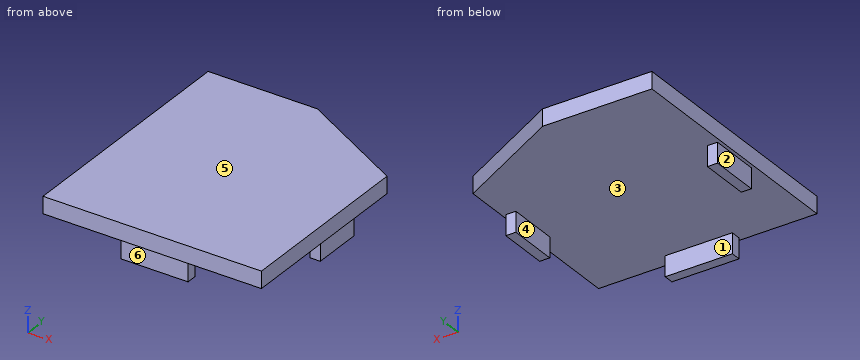
Autodesk Inventor part; units mm, degrees
ref_plane "YZ Plane" through (0, 0, 0) normal (1, 0, 0) x (0, 1, 0)
ref_plane "XZ Plane" through (0, 0, 0) normal (0, 1, 0) x (-1, 0, 0)
ref_plane "XY Plane" through (0, 0, 0) normal (0, 0, 1) x (1, 0, 0)
sketch "Sketch1" plane through (0, 0, 0) normal (0, 0, 1) x (1, 0, 0)
  line L0 (0, 175.2) -> (0, -29.2)
  line L1 (-91, 0) -> (91, 0)
  line L2 (0, 0) -> (-65, 0)
  line L3 (-65, 0) -> (-65, 146)
  line L4 (0, 0) -> (65, 0)
  line L5 (65, 0) -> (65, 111)
  line L6 (-65, 146) -> (0, 146)
  line L7 (0, 146) -> (65, 111)
  dimension "d0" = 65
  dimension "d1" = 146
  dimension "d2" = 65
  dimension "d3" = 111
  dimension "d4" = 65
extrude "Extrusion1" add sketch "Sketch1" along normal blind 10
sketch "Sketch2" plane through (0, 0, 0) normal (0, 0, -1) x (-1, 0, 0)
  line L0 (0, -29.2) -> (0, 175.2)
  line L1 (-91, 0) -> (91, 0)
  line L2 (65, 146) -> (65, 0)
  line L3 (0, 146) -> (65, 146)
  line L4 (-65, 111) -> (0, 146)
  line L5 (-65, 0) -> (-65, 111)
  line L6 (65, 0) -> (-65, 0)
  line L7 (-65, 0) -> (-55, 0)
  line L8 (-55, 0) -> (-55, 116.3846)
  line L9 (65, 0) -> (65, 10)
  line L10 (65, 10) -> (-65, 10)
  line L11 (65, 0) -> (55, 0)
  line L12 (55, 0) -> (55, 146)
  line L13 (-65, 0) -> (-65, 70)
  line L14 (-65, 70) -> (-63, 70)
  line L15 (-63, 70) -> (-63, 85)
  line L16 (-63, 85) -> (-57, 85)
  line L17 (-57, 85) -> (-57, 55)
  line L18 (-57, 55) -> (-63, 55)
  line L19 (-63, 55) -> (-63, 70)
  line L20 (65, 0) -> (65, 70)
  line L21 (65, 70) -> (63, 70)
  line L22 (63, 70) -> (63, 85)
  line L23 (63, 85) -> (57, 85)
  line L24 (57, 85) -> (57, 55)
  line L25 (57, 55) -> (63, 55)
  line L26 (63, 70) -> (63, 55)
  line L27 (0, 0) -> (0, 2)
  line L28 (0, 2) -> (-20, 2)
  line L29 (-20, 2) -> (-20, 8)
  line L30 (-20, 8) -> (20, 8)
  line L31 (20, 8) -> (20, 2)
  line L32 (20, 2) -> (0, 2)
  dimension "d7" = 10
  dimension "d8" = 10
  dimension "d9" = 10
  dimension "d10" = 70
  dimension "d11" = 2
  dimension "d12" = 15
  dimension "d13" = 6
  dimension "d14" = 30
  dimension "d15" = 70
  dimension "d16" = 2
  dimension "d17" = 15
  dimension "d18" = 6
  dimension "d19" = 30
  dimension "d20" = 2
  dimension "d21" = 20
  dimension "d22" = 6
  dimension "d23" = 40
extrude "Extrusion2" add sketch "Sketch2" along normal blind 12 contours L28 L29 L30 L0 | L0 L30 L31 L32 | L15 L16 L17 L18 L19 | L26 L25 L24 L23 L22
properties part number "Afsluitklep"
Could you check a few things on this model? Use its own coordinates, in mm. Face numbers are marked on the shaded views. A direction names the side the tool comes from. Give positions to 0.01 mm unless a question says otherwise; leave off trailing zeros. Loops run counter-clockwise (first coordinate to the right, second up) from the corner with the lowest first, then second, coordinate; pieces in that order, holes last. Notation, with made-up numbers: (47, 27.5) - (98, 27.5) arc R11 ccw to (98, 39.5) - close; hole circle Ø3 at (6.25, -23). An arc over 180 degrees is marked (long way). Answer in a Markdown table with one row per item. Add a question column.
Q1. If we section it at C-C (y = 73.5): List the corners of the cut face in (x, z) for me.
Q2. For pin 1 (1.5 mm diameter, centred on x = 29, y = 68.5, fed in from -Z); pin 2 (6 mm diameter, centred on y = 63.5, z = -6, fed in from -X); pin 3 (6 mm diameter, centred on y = 72.5, z = -5.5, fed in from +X); pin 4 (2 mm diameter, centred on x = -24, z = 3, fed in from -Y), each with a flat end and sliding along its axis, tell me the tip position at first contact or that it passes through.
Q3. We'd pull the mould along X, two halves only. Please class the marked faces 1, 2 and 3: +X half, -X half, draft (parallel to the pull), parting line (faces both ways), or undercut.
Q4. Please list where these lines run through material, in increasing order: L1, parallel to Z at x = 1, y = 62.5; L2, parallel to X at y = 77.5, z = -10.5; L3, parallel to Y at x = 3, z = -5.5. Write a range as from..to.
Q5. If we section it at A-A (z = -5.25): List the corners of the cut face in (x, y) for me, plus the area to 3 significant figures.
Q6. If we section it at D-D (z = 2.75): List the corners of the cut face in (x, y) for me, plus the area to 3 significant figures.
Q7. If we section it at B-B (x = -10.5): List the corners of the cut face in (y, z) for me, plus the area to 3 significant figures.
Q8. Which directions (+Z, -Z, +X, -X, +Y, -Y) give clear straight access to the entire face, cutting with the end or side of a thin tool? Please do the marked faces 4, 5 and 6.
The answers:
| question | item | result |
|---|---|---|
| 1 | outline | (-65, 0) - (-63, 0) - (-63, -12) - (-57, -12) - (-57, 0) - (57, 0) - (57, -12) - (63, -12) - (63, 0) - (65, 0) - (65, 10) - (-65, 10) - close |
| 2 | pin 1 | stops at z = 0 |
| 2 | pin 2 | stops at x = -63 |
| 2 | pin 3 | stops at x = 63 |
| 2 | pin 4 | stops at y = 0 |
| 3 | face 1 | draft |
| 3 | face 2 | -X half |
| 3 | face 3 | undercut |
| 4 | L1 | z = 0..10 |
| 4 | L2 | x = -63..-57, 57..63 |
| 4 | L3 | y = 2..8 |
| 5 | outline | (-63, 55) - (-57, 55) - (-57, 85) - (-63, 85) - close; (-20, 2) - (20, 2) - (20, 8) - (-20, 8) - close; (57, 55) - (63, 55) - (63, 85) - (57, 85) - close |
| 5 | area | 600 mm^2 |
| 6 | outline | (-65, 0) - (65, 0) - (65, 111) - (0, 146) - (-65, 146) - close |
| 6 | area | 17,800 mm^2 |
| 7 | outline | (0, 0) - (2, 0) - (2, -12) - (8, -12) - (8, 0) - (146, 0) - (146, 10) - (0, 10) - close |
| 7 | area | 1,530 mm^2 |
| 8 | face 4 | -Z, +Y, -Y |
| 8 | face 5 | +Z, +X, -X, +Y, -Y |
| 8 | face 6 | -Z, +X, -X, -Y |
